Geometry: see drawing. Coordinates: mm, zero at the bounding-box minimum. Round coordinates to 2 decimals unless told otherwise and drop trailing zeros. Order: outer loops, then holes, each group sorted by start corner. A loop starts at its lowest first (then second) coordinate and runs counter-clockwise, first axis right, second up. Notation, with made-up numbers: (27, 2) -> (45, 2) arc R9 ccw to (45, 15) -> close; hole circle Ø2 at (20, -31.75). An arc over 180 degrees is marked (long way). One line per item, written item: value. Start each with the question number.
1) Section B-B (y = 26.5). Return the cut outline in (x, z).
2) Ray query, L1, parallel to X at y = 27, z = 3.25; L2, parallel to Z at x = 41, y = 25.75; L3, parallel to Y at x = 5, z = 2.5 (1 decimal). Return the intervals inside material, ascending.
3) Section A-A (x = 35). Return the cut outline in (y, z) (1 decimal).
4) Section C-C (z = 3.1). State how many separate pieces and enclosed holes the cut face has, and give its area (3 significant figures).
5) Pin query (flat end, axial travel): P1, Ø1, axis at x = 17, z = 2.5, coming from the -Y side; P2, Ø3, axis at x = 16, z = 3.1, coming from the +Y side (1 decimal). Return the tip coordinate at first contact, or that it passes through.
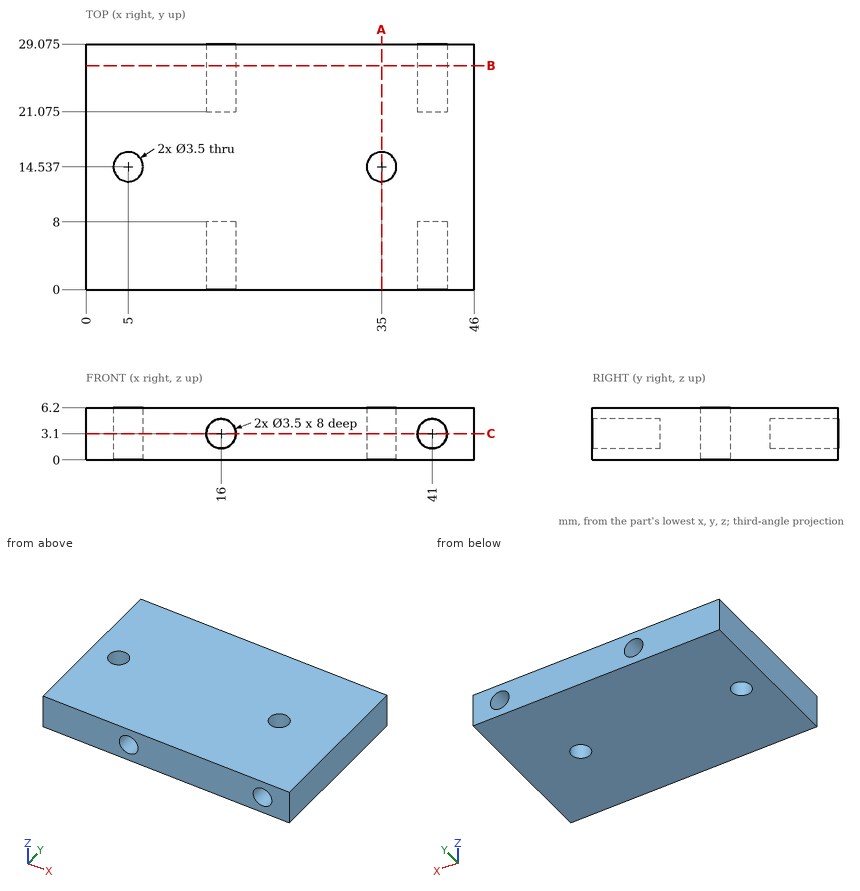
Findings:
1. outline: (0, 0) -> (46, 0) -> (46, 6.2) -> (0, 6.2) -> close; hole circle Ø3.5 at (16, 3.1); hole circle Ø3.5 at (41, 3.1)
2. L1: 0 to 14.26, 17.74 to 39.26, 42.74 to 46
2. L2: 0 to 1.35, 4.85 to 6.2
2. L3: 0 to 12.8, 16.3 to 29.1
3. outline: (0, 0) -> (12.8, 0) -> (12.8, 6.2) -> (0, 6.2) -> close; (16.3, 0) -> (29.1, 0) -> (29.1, 6.2) -> (16.3, 6.2) -> close
4. separate pieces: 1
4. enclosed holes: 2
4. area: 1,210 mm2
5. P1: y = 8
5. P2: y = 21.1
